Geometry: see drawing. Coordinates: mm, zero at the bounding-box minimum. Coordinates: 2 decimals unless noted, no trailing zeros. Loops run counter-clockwise (first coordinate to the right, second up) from the corner with the lowest first, then second, coordinate; pieces in that order, holes last. Notation, with made-up numbers: (12, 38.5) - (32, 38.5) arc R22 cw to (32, 50.5) - close; hole circle Ø1 at (-6, -33). An arc over 180 degrees is marked (long way). Use a Markdown table: item, result. Add a question column.
1. Section query A-A on z = 17.5. Return the cut outline in (x, y), then the cut area to 3 significant figures.
2. Section query B-B on y = 2.35. Return the cut outline in (x, z).
3. Section query C-C on x = 28.5. Return the cut outline in (y, z), then the cut area to 3 significant figures.
4. Ray query, L1, parallel to Z at x = 8.5, y = 1.75; L2, parallel to X at y = 2.8, z = 28.5; L3, parallel to X at y = 1.2, z = 17.5. Return the intervals inside material, ascending. Write a range as [from, to].
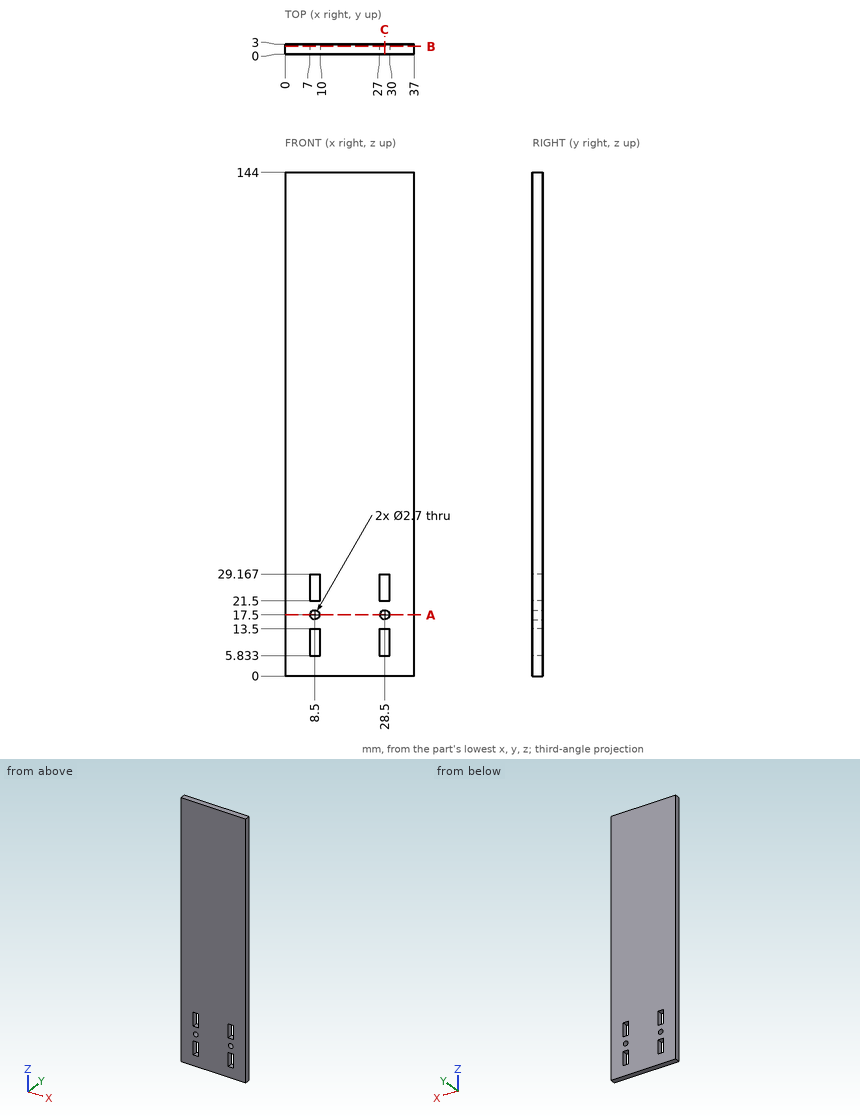
Resolved:
| question | item | result |
|---|---|---|
| 1 | outline | (0, 0) - (7.15, 0) - (7.15, 3) - (0, 3) - close; (9.85, 0) - (27.15, 0) - (27.15, 3) - (9.85, 3) - close; (29.85, 0) - (37, 0) - (37, 3) - (29.85, 3) - close |
| 1 | area | 94.8 mm² |
| 2 | outline | (0, 0) - (37, 0) - (37, 144) - (0, 144) - close; hole (7, 5.83) - (10, 5.83) - (10, 13.5) - (7, 13.5) - close; hole (7, 21.5) - (10, 21.5) - (10, 29.17) - (7, 29.17) - close; hole circle Ø2.7 at (8.5, 17.5); hole (27, 5.83) - (30, 5.83) - (30, 13.5) - (27, 13.5) - close; hole (27, 21.5) - (30, 21.5) - (30, 29.17) - (27, 29.17) - close; hole circle Ø2.7 at (28.5, 17.5) |
| 3 | outline | (0, 0) - (3, 0) - (3, 5.83) - (0, 5.83) - close; (0, 13.5) - (3, 13.5) - (3, 16.15) - (0, 16.15) - close; (0, 18.85) - (3, 18.85) - (3, 21.5) - (0, 21.5) - close; (0, 29.17) - (3, 29.17) - (3, 144) - (0, 144) - close |
| 3 | area | 378 mm² |
| 4 | L1 | [0, 5.83], [13.5, 16.15], [18.85, 21.5], [29.17, 144] |
| 4 | L2 | [0, 7], [10, 27], [30, 37] |
| 4 | L3 | [0, 7.15], [9.85, 27.15], [29.85, 37] |
